Check sheet for the drawn part. Datum: minimum x, y, z corner. Units: mm. Round coordinates to 2 decimals unless told otherwise and drop trailing zeros. Order: outer loops, then holes, each group sorted by start corner. A loop starts at its lowest first (then second) coordinate and runs counter-clockwise, first axis right, second up.
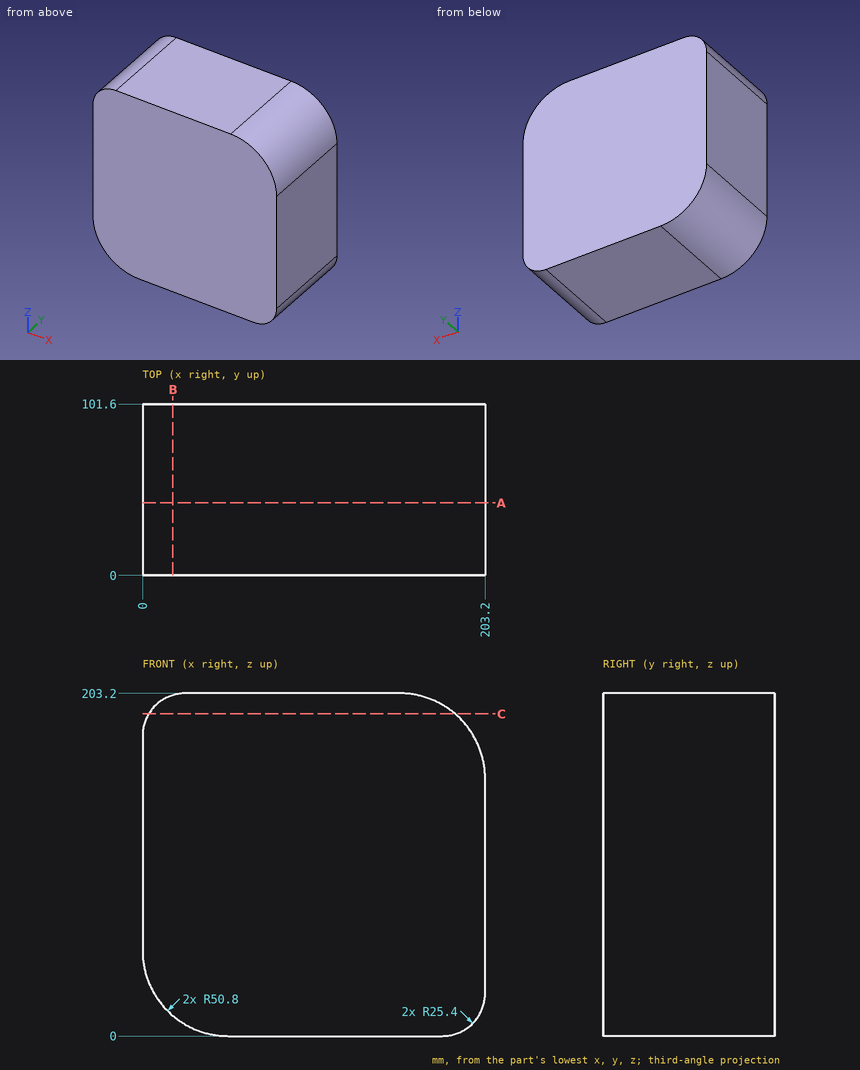
(1) Material ranges on line 1 (X direction, y = 57.5, z = 50.5); line 2 (X direction, y = 51, z = 42); line 3 (Z direction, x = 36, y = 78), recorded low to high.
Returned:
line 1: x = 0 to 203.2
line 2: x = 0.77 to 203.2
line 3: z = 2.2 to 203.2
(2) Sectioned sample at A-A, the plane y = 43. Record the cut outline in (x, z).
Returned:
outline: (0, 50.8) arc R50.8 ccw to (50.8, 0) - (177.8, 0) arc R25.4 ccw to (203.2, 25.4) - (203.2, 152.4) arc R50.8 ccw to (152.4, 203.2) - (25.4, 203.2) arc R25.4 ccw to (0, 177.8) - close
(3) Sectioned sample at B-B, the plane x = 18. Record the cut outline in (y, z).
Returned:
outline: (0, 12.01) - (101.6, 12.01) - (101.6, 202.1) - (0, 202.1) - close
(4) Sectioned sample at C-C, the plane z = 191. Record the cut outline in (x, y).
Returned:
outline: (3.7, 0) - (185.43, 0) - (185.43, 101.6) - (3.7, 101.6) - close
